```python
from build123d import *

# Parameters (mm, degrees)
SZKIC1_R                    = 3.5
DODANIE_WYCI_GNI_CIE1_DEPTH = 9.5
SZKIC2_R                    = 1.9
WYTNIJ_WYCI_GNI_CIE1_DEPTH  = 3.5
SZKIC3_R                    = 2
DODANIE_WYCI_GNI_CIE2_DEPTH = 1.6
WYTNIJ_WYCI_GNI_CIE2_START  = -0.6
SZKIC4_R                    = 2.15
WYTNIJ_WYCI_GNI_CIE2_DEPTH  = 0.6
SZKIC5_R                    = 1
WYTNIJ_WYCI_GNI_CIE3_DEPTH  = 31.6
SZKIC6_R                    = 3.5
SZKIC6_R_2                  = 2.75
WYTNIJ_WYCI_GNI_CIE4_DEPTH  = 0.6
WYTNIJ_WYCI_GNI_CIE5_DEPTH  = 10


with BuildPart() as part:
    # Szkic1 → Dodanie-wyciągnięcie1 (new body)
    with BuildSketch(Plane(origin=(0, 0, 0), x_dir=(1, 0, 0), z_dir=(0, 1, 0))):
        Circle(SZKIC1_R)
    extrude(amount=DODANIE_WYCI_GNI_CIE1_DEPTH)

    # Szkic2 → Wytnij-wyciągnięcie1 (cut)
    with BuildSketch(Plane.XZ):
        Circle(SZKIC2_R)
    extrude(amount=-WYTNIJ_WYCI_GNI_CIE1_DEPTH, mode=Mode.SUBTRACT)

    # Szkic3 → Dodanie-wyciągnięcie2 (add)
    with BuildSketch(Plane(origin=(0, 8.9, 0), x_dir=(1, 0, 0), z_dir=(0, 1, 0))):
        with Locations((-8.95, 0)):
            Circle(SZKIC3_R)
        with BuildLine():
            Line((-2, 2), (-8.95, 2))
            ThreePointArc((-8.95, 2), (-7.535786438, 1.414213562), (-6.95, 0))
            ThreePointArc((-6.95, 0), (-7.535786438, -1.414213562), (-8.95, -2))
            Line((-8.95, -2), (-2, -2))
            Line((-2, -2), (-2, 2))
        make_face()
        with Locations((0, 7)):
            Circle(SZKIC3_R)
        with BuildLine():
            Line((-2, 7), (-2, 2))
            Line((-2, 2), (0, 2))
            Line((0, 2), (2, 2))
            Line((2, 2), (2, 7))
            ThreePointArc((2, 7), (0, 5), (-2, 7))
        make_face()
        with BuildLine():
            Line((8.95, 2), (2, 2))
            Line((2, 2), (2, 0))
            Line((2, 0), (2, -2))
            Line((2, -2), (8.95, -2))
            ThreePointArc((8.95, -2), (6.95, 0), (8.95, 2))
        make_face()
        with Locations((8.95, 0)):
            Circle(SZKIC3_R)
        with Locations((0, -7)):
            Circle(SZKIC3_R)
        with BuildLine():
            Line((2, -2), (-2, -2))
            Line((-2, -2), (-2, -7))
            ThreePointArc((-2, -7), (0, -5), (2, -7))
            Line((2, -7), (2, -2))
        make_face()
    extrude(amount=-DODANIE_WYCI_GNI_CIE2_DEPTH)

    # Szkic4 → Wytnij-wyciągnięcie2 (cut)
    with BuildSketch(Plane(origin=(0, 9.5, 0), x_dir=(1, 0, 0), z_dir=(0, 1, 0)).offset(WYTNIJ_WYCI_GNI_CIE2_START)):
        Circle(SZKIC4_R)
    extrude(amount=WYTNIJ_WYCI_GNI_CIE2_DEPTH, mode=Mode.SUBTRACT)

    # Szkic5 → Wytnij-wyciągnięcie3 (cut)
    with BuildSketch(Plane(origin=(0, 8.9, 0), x_dir=(1, 0, 0), z_dir=(0, 1, 0))):
        Circle(SZKIC5_R)
    extrude(amount=-WYTNIJ_WYCI_GNI_CIE3_DEPTH, mode=Mode.SUBTRACT)

    # Szkic6 → Wytnij-wyciągnięcie4 (cut)
    with BuildSketch(Plane(origin=(0, 9.5, 0), x_dir=(1, 0, 0), z_dir=(0, 1, 0))):
        Circle(SZKIC6_R)
        Circle(SZKIC6_R_2, mode=Mode.SUBTRACT)
    extrude(amount=-WYTNIJ_WYCI_GNI_CIE4_DEPTH, mode=Mode.SUBTRACT)

    # Szkic7 → Wytnij-wyciągnięcie5 (cut)
    with BuildSketch(Plane.XZ.offset(-7.3)):
        with BuildLine():
            ThreePointArc((-2, -7), (0, -9), (2, -7))
            Line((2, -7), (2, -2.872281323))
            ThreePointArc((2, -2.872281323), (0, -3.5), (-2, -2.872281323))
            Line((-2, -2.872281323), (-2, -7))
        make_face()
        with BuildLine():
            Line((2, -11.805294156), (2, -7))
            ThreePointArc((2, -7), (0, -9), (-2, -7))
            Line((-2, -7), (-2, -2.872281323))
            ThreePointArc((-2, -2.872281323), (-2.872281323, 2), (2, 2.872281323))
            Line((2, 2.872281323), (2, 7))
            Line((2, 7), (2, 11.668395205))
            Line((2, 11.668395205), (-21.006020829, 11.668395205))
            Line((-21.006020829, 11.668395205), (-21.006020829, -11.805294156))
            Line((-21.006020829, -11.805294156), (2, -11.805294156))
        make_face()
    extrude(amount=-WYTNIJ_WYCI_GNI_CIE5_DEPTH, mode=Mode.SUBTRACT)


solid = part.part
```
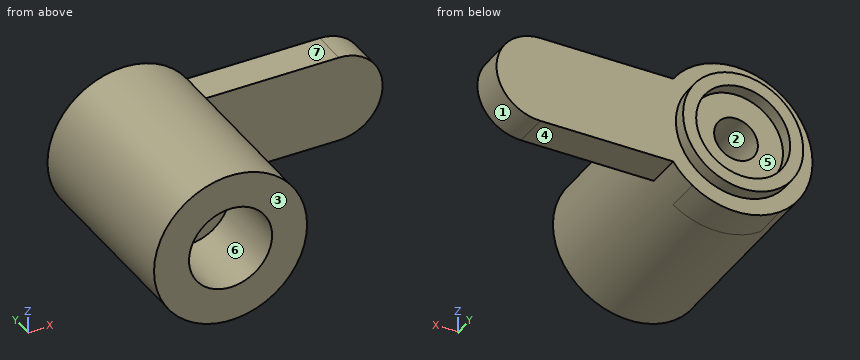
Part model, mm, in its own coordinate system. Face numbers are marked on the shaded views. A direction names the side the tool comes from. Round coordinates to 2 decimals unless told otherwise and drop trailing zeros. Write each loop counter-clockwise with the first axis right and the second up, starting at its lowest first coordinate (ties: lowest second). Pieces come first, ordered by that corner, then holes. Notation, with made-up numbers: M 7,65.25 L 45,65.25 A13 ccw 45,86.25 Z; hole C 18.5,25.25 d3. An arc over 180 degrees is marked long. Answer as CSV lines item,"result". Start each with the question number.
1) Band-saw the part on C-C (y = 8.5). List the corners of the cut face in (x, z), then the cut area to 3 significant figures.
2) Drop flat-ended pins along their axis: pin 1 (1.9 mm diameter, centred on x = 0, z = 0.5, fed in from -Y); pin 2 (0.8 mm diameter, centred on x = 4.5, y = 8, fed in from +Z); pin 3 (1.8 mm diameter, centred on x = 0, z = 0, fed in from +Y); pin 4 (4 mm diameter, centred on y = 1.5, z = 2.5, fed in from -X). Give the stop position or say it passes through.
3) Band-saw the part on B-B (z = 0). List the corners of the cut face in (x, y).
4) Band-saw the part on A-A (x = 0). List the corners of the cut face in (y, z).
5) Band-saw the part on D-D (x = 8). List the corners of the cut face in (y, z), then the cut area to 3 significant figures.
6) Mould opens along Z. For the marked faces 1, 2 and 3 say: +Z half, -Z half, draft (parallel to the pull), parting line (faces both ways), or undercut.
7) Which spindle directions (+Z, -Z, +X, -X, +Y, -Y) get a long thin tool onto all of the face, cutting with end or side? Do the marked faces 4, 5, 6 and 7. Say none if no direction does.
8) Drill centre lines: L1, parallel to Z at x = 0, y = 5.8; L2, parallel to X at y = 9.3, z = 0. Where is each one in solid material? Low to high.
Worked out:
1,outline,"M 2.87,-2 L 8.95,-2 A2 ccw 8.95,2 L 2.87,2 A3.5 ccw long Z; hole C 0,0 d2"
1,area,"64.2 mm²"
2,pin 1,"y = 3.5"
2,pin 2,"z = 2"
2,pin 3,"through"
2,pin 4,"x = -3.46"
3,outline,"M -3.5,0 L -1.9,0 L -1.9,3.5 L -1,3.5 L -1,8.9 L -2.15,8.9 L -2.15,9.5 L -2.75,9.5 L -2.75,8.9 L -3.5,8.9 Z; M 1,3.5 L 1.9,3.5 L 1.9,0 L 3.5,0 L 3.5,7.3 L 10.95,7.3 L 10.95,8.9 L 2.75,8.9 L 2.75,9.5 L 2.15,9.5 L 2.15,8.9 L 1,8.9 Z"
4,outline,"M 0,-3.5 L 8.9,-3.5 L 8.9,-2.75 L 9.5,-2.75 L 9.5,-2.15 L 8.9,-2.15 L 8.9,-1 L 3.5,-1 L 3.5,-1.9 L 0,-1.9 Z; M 0,1.9 L 3.5,1.9 L 3.5,1 L 8.9,1 L 8.9,2.15 L 9.5,2.15 L 9.5,2.75 L 8.9,2.75 L 8.9,3.5 L 0,3.5 Z"
5,outline,"M 7.3,-2 L 8.9,-2 L 8.9,2 L 7.3,2 Z"
5,area,"6.40 mm²"
6,face 1,"parting line"
6,face 2,"undercut"
6,face 3,"draft"
7,face 4,"-Z, +X, +Y, -Y"
7,face 5,"+Y"
7,face 6,"-Y"
7,face 7,"+Z, +X, +Y, -Y"
8,L1,"-3.5 to -1, 1 to 3.5"
8,L2,"-2.75 to -2.15, 2.15 to 2.75"
